The listing builds one solid part. Answer for the finished solid, in the listing's coordinates (mm). A direction names the side the tool comes from. Give positions to 0.01 mm unless a question says otherwise; leave off trailing zeros. Order: outer loops, then holes, each group sorted by start corner. A loop starts at its lowest first (then second) coordinate and runs counter-clockwise, first axis right, second up.
```python
from build123d import *

# Parameters (mm, degrees)
F0_W     = 17
F0_H     = 8
F1_DEPTH = 11
F3_DEPTH = 8
F5_D     = 3.5


with BuildPart() as f1:
    # F0 (on Front) → F1 (new body)
    with BuildSketch(Plane.XZ):
        with Locations((8.5, 4)):
            Rectangle(F0_W, F0_H)
    extrude(amount=F1_DEPTH)

    # F2 (on face) → F3 (join)
    with BuildSketch(Plane.XY.offset(8)):
        Polygon((0, -11), (2.6, -11), (2.6, -2.6), (17, -2.6), (17, 0), (0, 0), align=None)
    extrude(amount=F3_DEPTH)

    # F5 (through all)
    with Locations(Plane.YZ.offset(2.6)):
        with Locations((-6.8, 12.1)):
            Hole(F5_D / 2)


solid = f1.part
```
1) For a pull along Z with two mould halves and no side action, classify faces 3 (the cylindrical face through (1.28, -5.41, 11.04)), 4 (the flat face through (2.6, -7, 10)), 5 (the flat face through (8, -5, 0)), 6 (the flat face through (10, -7, 8)) as +Z half, -Z half, draft (parallel to the pull), parting line (faces both ways), or undercut.
Geometry says:
face 3: undercut
face 4: draft
face 5: -Z half
face 6: +Z half
2) Find section B-B (z = 12.1). Write down the section's boundary in (x, y).
Geometry says:
outline: (0, -11) - (2.6, -11) - (2.6, -8.55) - (0, -8.55) - close; (0, -5.05) - (2.6, -5.05) - (2.6, -2.6) - (17, -2.6) - (17, 0) - (0, 0) - close
3) Find section A-A (y = -6.8). Write down the section's boundary in (x, z).
Geometry says:
outline: (0, 0) - (17, 0) - (17, 8) - (2.6, 8) - (2.6, 10.35) - (0, 10.35) - close; (0, 13.85) - (2.6, 13.85) - (2.6, 16) - (0, 16) - close
4) Find section D-D (z = 9.75). Write down the section's boundary in (x, y), then the cut area to 3 significant figures.
Geometry says:
outline: (0, -11) - (2.6, -11) - (2.6, -2.6) - (17, -2.6) - (17, 0) - (0, 0) - close
area: 66.0 mm2
5) Straight lines are drawn through the part: probe 1 along Z at (x, y) = (1.7, -6.8); probe 2 along Z at (x, y) = (14, -5.25); probe 3 along Y at (x, z) = (5.75, 11.5). For each, find the intervals that lie inside material, in ascending order.
Geometry says:
probe 1: z = 0 to 10.35, 13.85 to 16
probe 2: z = 0 to 8
probe 3: y = -2.6 to 0
6) A tool of negligible diameter and unlimited length cuts with its end or side. For faces 1 (the flat face through (9, 0, 8)), 2 (the flat face through (10, -2.6, 12)), from which of +Z, -Z, +X, -X, +Y, -Y can it reach the whole face along a straight path? Write none if from no direction.
Geometry says:
face 1: +Z, -Z, +X, -X, +Y
face 2: +Z, +X, -Y
7) Find section C-C (x = 1.75). Write down the section's boundary in (y, z), then the cut area to 3 significant figures.
Geometry says:
outline: (-11, 0) - (0, 0) - (0, 16) - (-11, 16) - close; hole circle Ø3.5 at (-6.8, 12.1)
area: 166 mm2
8) Given P1, Ø6.5, axis at x = 11, y = -6, coming from the +Z side, flat-ended and moving along its own axis, determine where the tip first touches the part or whether it passes through.
Geometry says:
P1: stops at z = 8
